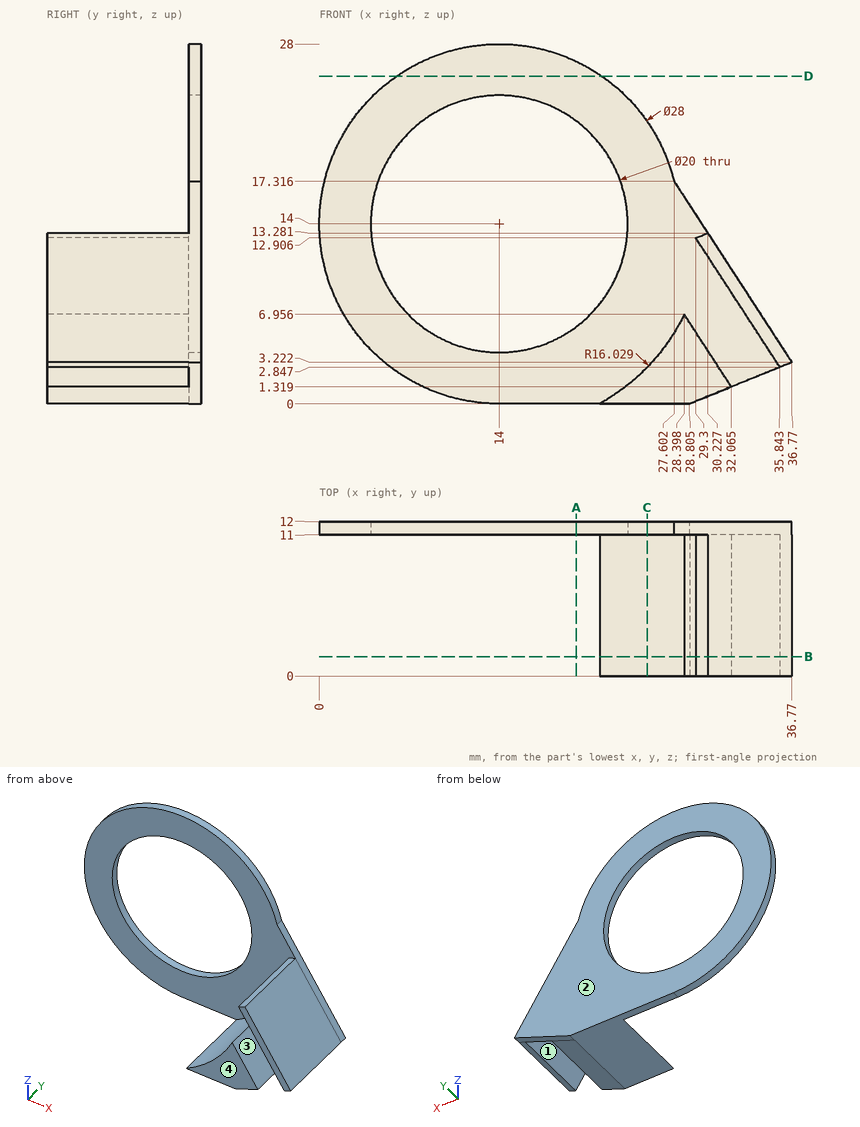
Part print with two shaded views. Sizes in mm from the minimum x, y, z corner. A direction names the side the tool comes from. Coordinates: 2 decimals unless noted, no trailing zeros. Order: outer loops, then holes, each group sorted by start corner. A loop starts at its lowest first (then second) coordinate and runs counter-clockwise, first axis right, second up. Notation, with made-up numbers: (88, 61) - (120, 61) arc R26 ccw to (120, 90) - close; hole circle Ø9 at (-10, 48). An arc over 180 degrees is marked (long way). Answer in a Markdown table with one row per item.
1. Slice it at B-B, the plane y = 1.5. List the corners of the cut face in (x, z) (1 decimal).
Answer:
| item | result |
|---|---|
| outline | (21.8, 0) - (28.8, 0) - (32.1, 1.3) - (28.4, 7) arc R16 cw to start; (29.3, 12.9) - (35.8, 2.8) - (36.8, 3.2) - (30.2, 13.3) - close |
2. Slice it at A-A, the plane x = 20. List the corners of the cut face in (y, z).
Answer:
| item | result |
|---|---|
| outline | (11, 0) - (12, 0) - (12, 6) - (11, 6) - close; (11, 22) - (12, 22) - (12, 26.65) - (11, 26.65) - close |
3. Pull direction X, two halves, no side cores. Call the marked faces 3 and 4: +X half, -X half, draft (parallel to the pull), parting line (faces both ways), or undercut.
Answer:
| item | result |
|---|---|
| face 3 | undercut |
| face 4 | draft |
4. Slice it at D-D, the plane z = 25.5. List the corners of the cut face in (x, y) (1 decimal).
Answer:
| item | result |
|---|---|
| outline | (6, 11) - (22, 11) - (22, 12) - (6, 12) - close |
5. 3-axis set-ups, long thin cutter, end or side, ignore diameter. For the marked faces 1 and 2: which of +Z, -Z, +X, -X, +Y, -Y reach the whole face in a straight line?
Answer:
| item | result |
|---|---|
| face 1 | -Y |
| face 2 | +Z, -Z, +X, -X, +Y |
6. Drill centre lines: L1, parallel to Y at x = 6, z = 7; L2, parallel to X at y = 11.45, z = 14; L3, parallel to X at y = 6, z = 5.75 (1 decimal). Where is each one in solid material? Low to high. Write a range as from..to.
Answer:
| item | result |
|---|---|
| L1 | 11..12 |
| L2 | 0..4, 24..29.76 |
| L3 | 27.7..29.2, 34..35.1 |
7. Flat gauge pins, fed straight in: P1, Ø4, axis at y = 4, z = 12.5, coming from the +X side (1 decimal); P2, Ø12, axis at x = 10, z = 8, coming from the -Y side; P3, Ø6, axis at y = 6, z = 15, coming from the +X side. Where does each tip first touch, or does it go through?
Answer:
| item | result |
|---|---|
| P1 | x = 32 |
| P2 | y = 11 |
| P3 | x = 31.06 |
8. Slice it at C-C, the plane x = 25.5. List the corners of the cut face in (y, z) (1 decimal).
Answer:
| item | result |
|---|---|
| outline | (0, 0) - (12, 0) - (12, 22) - (11, 22) - (11, 2.8) - (0, 2.8) - close |
